Source: CAD feature listing. Evaluate the final solid. Frame: model axes, mm. A direction names the side the tool comes from. Give positions to 0.01 mm unless a question says otherwise; leave off trailing zeros. Order: outer loops, then holes, each group sorted by start corner. A loop starts at its lowest first (then second) coordinate and runs counter-clockwise, first axis right, second up. Notation, with made-up numbers: M 26,63.25 L 67,63.25 A20 cw 67,95.25 Z; hole C 41,1 d1. An arc over 180 degrees is marked long. Answer in a Markdown table with one row per item. Add a question column.
(1) Material intervals for line 1 along Z through (x, y) = (6.5, 0.25); line 2 along X through (y, z) = (0, -7.25); line 3 along X through (y, z) = (8.5, -1), sorted ascending.
(2) Mould query, pull axis Y, two halves, no side actions, for faces 1 (the face through (18, 0, 0)), 2 (the face through (1, 1.25, 0)), 3 (the face through (3.62, -2.94, 9.34)). Classes: pulls with the +Y half, pulls with the -Y half, needs draft (parallel to the pull), parting line crosses it, or undercut.
(3) Section query B-B, the plane y = 0. Return loops of the section in (x, z), plus the area to 3 significant figures.
(4) Section query A-A, the plane z = 0. Return loops of the section in (x, y), plus the area to 3 significant figures.
(5) Set-up query: faces 4 (the face through (12, 0, -5)), 5 (the face through (0, 3, 0)), 6 (the face through (1, -1.25, 0)). Return all of +Z, -Z, +X, -X, +Y, -Y with unobstructed straight access to the full face (end or side cutting, diameter ignored); none if empty.
(6) Section query C-C, the plane x = 15.75. Return loops of the section in (y, z).
(7) Pin query (flat end, axial travel): P1, Ø2, axis at y = -7.5, z = 6.5, coming from the -X side; P2, Ø4, axis at x = 3.5, y = 1.5, coming from the +Z side; P3, Ø6, axis at x = 14.5, y = 2, coming from the -Z side. Return the tip coordinate at first contact, or that it passes through.
(8) Section query D-D, the plane x = 5. Return loops of the section in (y, z).
from build123d import *

# Parameters (mm, degrees)
FILLET2_R  = 3
SKETCH2_W  = 20
SKETCH2_H  = 2.5
SLOT_DEPTH = 2.4


with BuildPart() as part:
    # BodySke → Base-Revolve (revolve)
    with BuildSketch(Plane.XY, mode=Mode.PRIVATE) as base_revolve_sk:
        Polygon((6, 5), (6, 10), (0, 9.475068019), (0, 0), (18, 0), (18, 5), align=None)
    revolve(base_revolve_sk.sketch.rotate(Axis((-25.4, 0, 0), (1, 0, 0)), 90), axis=Axis((-25.4, 0, 0), (1, 0, 0)))  # turned: the seam where the file's is

    # Fillet2
    fillet2_edges = [part.edges().sort_by_distance(p)[0] for p in [
        (0, 0, -9.475068019),
    ]]
    fillet(fillet2_edges, radius=FILLET2_R)

    # Sketch2 → Slot (cut)
    with BuildSketch(Plane(origin=(0, 0, 0), x_dir=(0, 0, -1), z_dir=(1, 0, 0))):
        Rectangle(SKETCH2_W, SKETCH2_H)
    extrude(amount=SLOT_DEPTH, mode=Mode.SUBTRACT)


solid = part.part
Values follow:
| question | item | result |
|---|---|---|
| 1 | line 1 | z = -4.99 to 4.99 |
| 1 | line 2 | x = 2.4 to 6 |
| 1 | line 3 | x = 0.62 to 6 |
| 2 | face 1 | needs draft |
| 2 | face 2 | undercut |
| 2 | face 3 | parting line crosses it |
| 3 | outline | M 2.4,-9.67 A3 ccw 2.74,-9.71 L 6,-10 L 6,-5 L 18,-5 L 18,5 L 6,5 L 6,10 L 2.74,9.71 A3 ccw 2.4,9.67 Z |
| 3 | area | 191 mm² |
| 4 | outline | M 0,-6.73 A3 ccw 2.74,-9.71 L 6,-10 L 6,-5 L 18,-5 L 18,5 L 6,5 L 6,10 L 2.74,9.71 A3 ccw 0,6.73 L 0,1.25 L 2.4,1.25 L 2.4,-1.25 L 0,-1.25 Z |
| 4 | area | 228 mm² |
| 5 | face 4 | +X |
| 5 | face 5 | +Z, -Z, -X, +Y, -Y |
| 5 | face 6 | +Z, -Z, -X |
| 6 | outline | C 0,0 d10 |
| 7 | P1 | stops at x = 0.96 |
| 7 | P2 | stops at z = 9.92 |
| 7 | P3 | stops at z = -5 |
| 8 | outline | C 0,0 d19.83 |
